Study the drawing (mm; zero at the part's minimum x, y, z) and answer. A direction names the side the tool comes from. Round coordinates to 2 decimals unless told otherwise and drop trailing zeros. Loops run counter-clockwise (first coordinate to the right, second up) from the corner with the lowest first, then second, coordinate; pieces in that order, holes last. Notation, with made-up numbers: (-24, 82.5) - (-1, 82.5) arc R29 ccw to (-1, 120.5) - close; hole circle Ø7 at (-14.75, -20.5). An arc over 180 degrees is marked (long way). Use CSV: the item, a comma, the result in double quotes. Start each with the question number.
1. Find section D-D (y = 17). Give the vertices of the cut face in (x, z), and give its area (3 significant figures).
2. Find section A-A (z = 28). Give the vertices of the cut face in (x, y), and give its area (3 significant figures).
3. Find section C-C (y = 8.25). State how many separate pieces and enclosed holes the cut face has, and give its area (3 significant figures).
4. A tool of negligible diameter and unlimited length cuts with its end or side. For the marked faces 4, 5 and 6, from which of +Z, -Z, +X, -X, +Y, -Y can it reach the whole face along a straight path? Write none if from no direction.
5. Determine the mould class of the marked faces 1, 2 and 3 for opening direction X: +X half, -X half, draft (parallel to the pull), parting line (faces both ways), or undercut.
6. Consider line 1 along Y through (x, z) = (87.5, 13.5); line 2 along Y through (x, z) = (7.5, 30.75); line 3 along X through (y, z) = (8, 10). Determine where each line is inside the solid, lowest interval first.
7. Given pin 1 Ø5 at (x, y) = (55, 26) entering from +Z; pin 2 Ø4.5 at (x, y) = (85.5, 42.5) entering from +Z; pin 3 Ø2.5 at (y, z) = (17, 33.62) entering from +X, each flat-ended and moving along its own axis, determine where each tip first touches the part or whether it passes through.
8. Find section B-B (x = 87.5). Give the vertices of the cut face in (y, z).
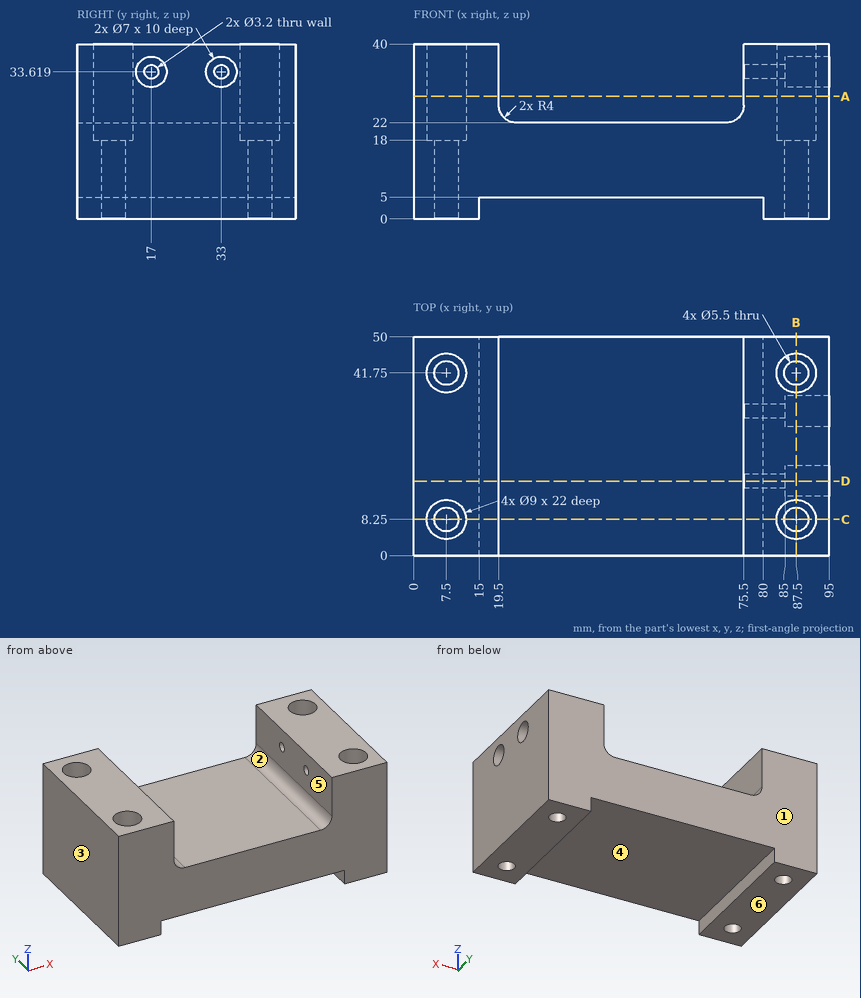
Filled sheet:
1,outline,"(0, 0) - (15, 0) - (15, 5) - (80, 5) - (80, 0) - (95, 0) - (95, 30.12) - (85, 30.12) - (85, 32.02) - (75.5, 32.02) - (75.5, 26) arc R4 cw to (71.5, 22) - (23.5, 22) arc R4 cw to (19.5, 26) - (19.5, 40) - (0, 40) - close; (75.5, 35.22) - (85, 35.22) - (85, 37.12) - (95, 37.12) - (95, 40) - (75.5, 40) - close"
1,area,"2,370 mm²"
2,outline,"(0, 0) - (19.5, 0) - (19.5, 50) - (0, 50) - close; (75.5, 0) - (95, 0) - (95, 50) - (75.5, 50) - close; hole circle Ø9 at (7.5, 8.25); hole circle Ø9 at (7.5, 41.75); hole circle Ø9 at (87.5, 8.25); hole circle Ø9 at (87.5, 41.75)"
2,area,"1,700 mm²"
3,separate pieces,"3"
3,enclosed holes,"0"
3,area,"1,880 mm²"
4,face 4,"-Z, +Y, -Y"
4,face 5,"+Z, +Y, -Y"
4,face 6,"-Z, +X, -X, +Y, -Y"
5,face 1,"draft"
5,face 2,"undercut"
5,face 3,"-X half"
6,line 1,"y = 0 to 5.5, 11 to 39, 44.5 to 50"
6,line 2,"y = 0 to 3.75, 12.75 to 37.25, 46.25 to 50"
6,line 3,"x = 0 to 4.76, 10.24 to 84.76, 90.24 to 95"
7,pin 1,"stops at z = 22"
7,pin 2,"stops at z = 18"
7,pin 3,"stops at x = 19.5"
8,outline,"(0, 0) - (5.5, 0) - (5.5, 18) - (3.75, 18) - (3.75, 40) - (0, 40) - close; (11, 0) - (39, 0) - (39, 18) - (37.25, 18) - (37.25, 40) - (12.75, 40) - (12.75, 18) - (11, 18) - close; (44.5, 0) - (50, 0) - (50, 40) - (46.25, 40) - (46.25, 18) - (44.5, 18) - close; hole circle Ø7 at (17, 33.62); hole circle Ø7 at (33, 33.62)"
